Geometry check sheet. Reference: the model listing, model coordinates, mm. A direction names the side the tool comes from. Coordinates: 2 decimals unless noted, no trailing zeros. Write each loop counter-clockwise with the first axis right and the second up, starting at its lowest first coordinate (ties: lowest second). Pieces come first, ordered by that corner, then holes. Notation, with made-up numbers: M 46.25,84.5 L 50.25,84.5 A21 cw 50.25,114.5 Z; hole C 81,-4.5 d5. An arc over 180 degrees is marked long. Write item = value, one per line. Start each with the question number.
```python
from build123d import *

# Parameters (mm, degrees)
CROQUIS1_W              = 50
CROQUIS1_H              = 50
SALIENTE_EXTRUIR1_DEPTH = 10
CROQUIS2_W              = 8
CROQUIS2_H              = 20
SALIENTE_EXTRUIR2_DEPTH = 20
CROQUIS3_R              = 3.5
CORTAR_EXTRUIR1_DEPTH   = 49.641546028
REDONDEO1_R             = 10
REDONDEO2_R             = 5
CHAFL_N1_SIZE           = 1


with BuildPart() as part:
    # Croquis1 → Saliente-Extruir1 (new body)
    with BuildSketch(Plane(origin=(0, 0, 0), x_dir=(1, 0, 0), z_dir=(0, 1, 0))):
        Rectangle(CROQUIS1_W, CROQUIS1_H)
    extrude(amount=SALIENTE_EXTRUIR1_DEPTH)

    # Croquis2 → Saliente-Extruir2 (add)
    with BuildSketch(Plane(origin=(0, 10, 0), x_dir=(1, 0, 0), z_dir=(0, 1, 0))):
        Rectangle(CROQUIS2_W, CROQUIS2_H)
    extrude(amount=SALIENTE_EXTRUIR2_DEPTH)

    # Croquis3 → Cortar-Extruir1 (cut, through all)
    with BuildSketch(Plane(origin=(4, 0, 0), x_dir=(0, 0, -1), z_dir=(1, 0, 0))):
        with Locations((0, 23)):
            Circle(CROQUIS3_R)
    extrude(amount=-CORTAR_EXTRUIR1_DEPTH, mode=Mode.SUBTRACT)

    # Redondeo1
    redondeo1_edges = [part.edges().sort_by_distance(p)[0] for p in [
        (0, 30, -10),
        (0, 30, 10),
    ]]
    fillet(redondeo1_edges, radius=REDONDEO1_R - 0.0001)  # a hair under: the kernel refuses the full size

    # Redondeo2
    redondeo2_edges = [part.edges().sort_by_distance(p)[0] for p in [
        (25, 5, 25),
        (-25, 5, 25),
        (-25, 5, -25),
        (25, 5, -25),
    ]]
    fillet(redondeo2_edges, radius=REDONDEO2_R)

    # Chaflán1
    chafl_n1_edges = [part.edges().sort_by_distance(p)[0] for p in [
        (-25, 10, 0),
        (0, 10, -25),
        (25, 10, 0),
        (0, 10, 25),
        (-23.535533906, 10, 23.535533906),
        (23.535533906, 10, 23.535533906),
        (23.535533906, 10, -23.535533906),
        (-23.535533906, 10, -23.535533906),
    ]]
    chamfer(chafl_n1_edges, length=CHAFL_N1_SIZE)


solid = part.part
```
Q1. Draft check along Z on faces 6 (the face through (4, 18, 0)), 7 (the face through (0.06, 26.47, 0.46)), 8 (the face through (0.06, 26.99, -7.15)). Enter one of: pulls with the +Z half, pulls with the -Z half, needs draft (parallel to the pull), parting line crosses it, or undercut.
Q2. Set-up check for faces 1 (the face through (0, 15, 10)), 2 (the face through (-22.996, 9.715, 23.063)), 3 (the face through (-4, 18, 0)), 4 (the face through (0, 15, -10)), 5 (the face through (25, 4, 0)): record each of +Z, -Z, +X, -X, +Y, -Y from which the full face is reachable in a straight line by a thin tool's end or side.
Q3. Gauge pin test, flat ends, axial feed: pin 1 (9 mm diameter, centred on x = 1.5, y = 15, fed in from -Z); pin 2 (10 mm diameter, centred on y = 18.5, z = -0.5, fed in from -X); pin 3 (5.5 mm diameter, centred on y = 23, z = 0, fed in from -X); pin 4 (2 mm diameter, centred on x = 4.5, y = 25, fed in from -Z). Record the tip position at first contact, or that the pin passes through.
Q4. Cross-section at B-B on z = 1. Enter the section's corners in (x, y).
Q5. Cross-section at D-D on x = 7.5. Enter the section's corners in (y, z).
Q6. Cross-section at C-C on z = -15.5. Enter the section's corners in (x, y), and give its area (3 significant figures).
Q7. Cross-section at A-A on y = 23. Enter the section's corners in (x, z), and give its area (3 significant figures).
Q8. Scan lines: L1, parallel to Y at x = 1, z = 0; L2, parallel to X at y = 15, z = -3.5; L3, parallel to Y at x = -4, z = -21.5. Record each from-to range of solid material in increasing order.
Values found:
q1.face_6 = needs draft
q1.face_7 = undercut
q1.face_8 = pulls with the -Z half
q2.face_1 = +Z, +X, -X, +Y
q2.face_2 = +Z, -X, +Y
q2.face_3 = +Z, -Z, -X, +Y
q2.face_4 = -Z, +X, -X, +Y
q2.face_5 = +Z, -Z, +X, +Y, -Y
q3.pin_1 = -10
q3.pin_2 = -4
q3.pin_3 = through
q3.pin_4 = -9.11
q4.outline = M -25,0 L 25,0 L 25,9 L 24,10 L 4,10 L 4,19.65 L -4,19.65 L -4,10 L -24,10 L -25,9 Z; M -4,26.35 L 4,26.35 L 4,29.95 L -4,29.95 Z
q5.outline = M 0,-25 L 9,-25 L 10,-24 L 10,24 L 9,25 L 0,25 Z
q6.outline = M -25,0 L 25,0 L 25,9 L 24,10 L -24,10 L -25,9 Z
q6.area = 499 mm²
q7.outline = M -4,-9.54 L 4,-9.54 L 4,-3.5 L -4,-3.5 Z; M -4,3.5 L 4,3.5 L 4,9.54 L -4,9.54 Z
q7.area = 96.6 mm²
q8.L1 = 0 to 19.5, 26.5 to 30
q8.L2 = -4 to 4
q8.L3 = 0 to 10
